Source: CAD feature listing. Evaluate the final solid. Frame: model axes, mm. Face numbers are marked on the shaded views. A direction names the side the tool comes from. Round coordinates to 2 decimals unless told otherwise and drop trailing zeros. Write each loop counter-clockwise with the first axis right and the second up, starting at its lowest first coordinate (ties: lowest second). Pieces come first, ordered by that corner, then holes. Notation, with made-up numbers: M -39,-40 L -14,-40 A15 ccw -14,-31 Z; hole C -4.75,-24 d11. An arc over 180 degrees is marked long. Answer in a Markdown table with one row per item.
from build123d import *

# Parameters (mm, degrees)
F0_W     = 68.6
F0_H     = 32.3
F1_DEPTH = 1
F2_W     = 68.6
F2_H     = 32.3
F2_W_2   = 64.6
F2_H_2   = 28.3
F3_DEPTH = 15.94
F4_W     = 13
F4_H     = 5.5
F5_DEPTH = 25


with BuildPart() as f1:
    # F0 (on Top) → F1 (new body)
    with BuildSketch(Plane.XY):
        with Locations((34.3, 16.15)):
            Rectangle(F0_W, F0_H)
    extrude(amount=F1_DEPTH)

    # F2 (on face) → F3 (join)
    with BuildSketch(Plane.XY.offset(1)):
        with Locations((34.3, 16.15)):
            Rectangle(F2_W, F2_H)
        with Locations((34.3, 16.15)):
            Rectangle(F2_W_2, F2_H_2, mode=Mode.SUBTRACT)
    extrude(amount=F3_DEPTH)

    # F4 (on face) → F5 (cut)
    with BuildSketch(Plane.YZ.offset(68.6)):
        with Locations((23.8, 14.19)):
            Rectangle(F4_W, F4_H)
    extrude(amount=-F5_DEPTH, mode=Mode.SUBTRACT)


solid = f1.part
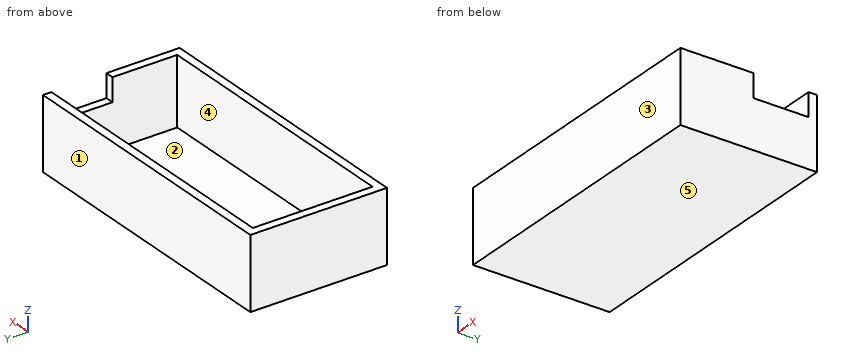
Q1. Pull-direction query (Y, two-part tool) for the marked faces 3, 4 and 5; classes: pulls with the +Y half, pulls with the -Y half, needs draft (parallel to the pull), parting line crosses it, or undercut.
Solutions:
| item | result |
|---|---|
| face 3 | pulls with the -Y half |
| face 4 | undercut |
| face 5 | needs draft |
Q2. Section A-A (z = 6). Return loops of the section in (x, y), and give its area (3 significant figures).
Solutions:
| item | result |
|---|---|
| outline | M 0,0 L 68.6,0 L 68.6,32.3 L 0,32.3 Z; hole M 2,2 L 66.6,2 L 66.6,30.3 L 2,30.3 Z |
| area | 388 mm2 |
Q3. Section C-C (x = 44). Return loops of the section in (y, z).
Solutions:
| item | result |
|---|---|
| outline | M 0,0 L 32.3,0 L 32.3,16.94 L 30.3,16.94 L 30.3,1 L 2,1 L 2,16.94 L 0,16.94 Z |
Q4. Contact query for flat-ended pins moving along their axis: pin 1 Ø1.6 at (x, y) = (67.5, 26) entering from +Z; pin 2 Ø14 at (x, y) = (29.5, 16.5) entering from +Z. Output: stop coordinate, or through.
Solutions:
| item | result |
|---|---|
| pin 1 | stops at z = 11.44 |
| pin 2 | stops at z = 1 |
Q5. Section D-D (z = 13). Return loops of the section in (x, y), and give its area (3 significant figures).
Solutions:
| item | result |
|---|---|
| outline | M 0,0 L 68.6,0 L 68.6,17.3 L 66.6,17.3 L 66.6,2 L 2,2 L 2,30.3 L 68.6,30.3 L 68.6,32.3 L 0,32.3 Z |
| area | 362 mm2 |
Q6. Material intervals for probe 1 along Y at (x, z) = (13, 3.5); probe 2 along X at (y, z) = (14, 8.75); probe 3 along Z at (x, y) = (48, 11.5), sorted ascending.
Solutions:
| item | result |
|---|---|
| probe 1 | y = 0 to 2, 30.3 to 32.3 |
| probe 2 | x = 0 to 2, 66.6 to 68.6 |
| probe 3 | z = 0 to 1 |
Q7. Section B-B (y = 16). Return loops of the section in (x, z).
Solutions:
| item | result |
|---|---|
| outline | M 0,0 L 68.6,0 L 68.6,16.94 L 66.6,16.94 L 66.6,1 L 2,1 L 2,16.94 L 0,16.94 Z |
Q8. Access query for the marked faces 1 and 2. Directions: +Z, -Z, +X, -X, +Y, -Y. A direction counts if a zero-diameter tool reaches every point of the face in a straight line with its end or side. Return the directions, or none.
Solutions:
| item | result |
|---|---|
| face 1 | +Z, -Z, +X, -X, +Y |
| face 2 | +Z |
